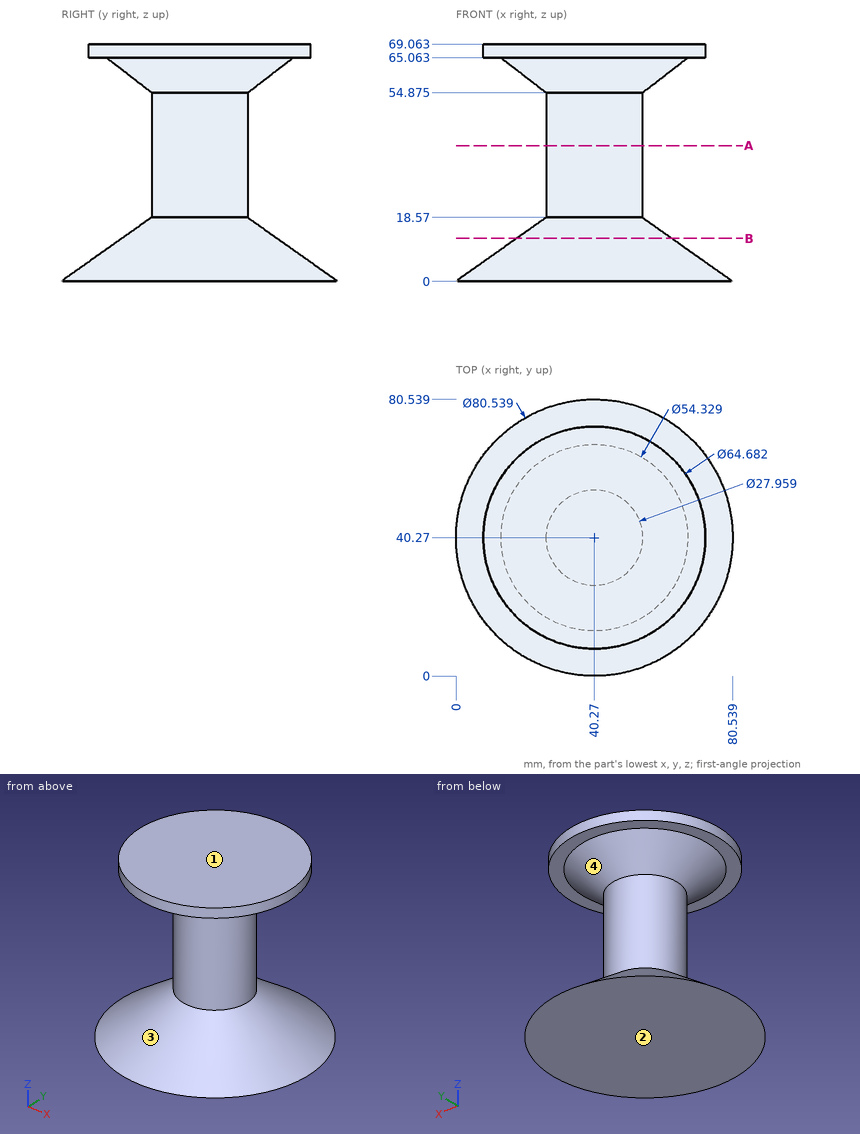
Here's the drawing with two shaded views (mm, measured from the low corner). I have some questions. Give positions to 0.01 mm unless a question says otherwise; leave off trailing zeros. Loops run counter-clockwise (first coordinate to the right, second up) from the corner with the lowest first, then second, coordinate; pieces in that order, holes last. Notation, with made-up numbers: M -23.75,21 L 32.25,21 A28 cw 32.25,53 Z; hole C 62,64.25 d1. An arc over 180 degrees is marked long. Use one line per item in the form item = value. Start each with the question number.
Q1. I need wall thicknesses on line 1 along Z through (x, y) = (24.5, 47.5) (1 decimal); line 2 along Z through (x, y) = (55, 56) (1 decimal); line 3 along Y through (x, z) = (38.5, 3). Which ranges of each line are inside material? Lowest first, please.
Q2. Will these pins go through, and if not, where does the flat tip stop? pin 1 Ø1 at (x, y) = (8.5, 49.5) entering from +Z; pin 2 Ø12 at (y, z) = (30.5, 38) entering from +X; pin 3 Ø12 at (x, z) = (56, 7) entering from -Y (1 decimal).
Q3. If we section it at B-B (z = 12.5): Write out the boundary of the cut face in (x, y).
Q4. If we section it at A-A (z = 39.5): Write out the boundary of the cut face in (x, y).
Q5. Thinking about a two-plate mould opening in Z: for the marked faces 1, 2, 3 and 4, which applies, +Z half, -Z half, draft (parallel to the pull), parting line (faces both ways), or undercut?
Taken from the geometry:
q1.line_1 = 0 to 16.2, 57.5 to 69.1
q1.line_2 = 0 to 13.2, 60.7 to 69.1
q1.line_3 = 4.29 to 76.25
q2.pin_1 = 5.43
q2.pin_2 = 53.73
q2.pin_3 = 4.4
q3.outline = C 40.27,40.27 d45.15
q4.outline = C 40.27,40.27 d27.96
q5.face_1 = +Z half
q5.face_2 = -Z half
q5.face_3 = undercut
q5.face_4 = undercut
